Read the model definition and answer for the solid it produces. Units are mm, in the model's axes. Coordinates: 2 decimals unless noted, no trailing zeros. Write each loop counter-clockwise with the first axis right and the second up, starting at its lowest first coordinate (ties: lowest second). Pieces come first, ordered by that corner, then holes. Notation, with made-up numbers: (20, 17.25) -> (36, 17.25) arc R19 ccw to (36, 45.25) -> close; hole circle Ø2 at (-13, 54.5). An arc over 180 degrees is marked (long way). Use CSV: the item, a comma, the result in double quotes.
from build123d import *

# Parameters (mm, degrees)
EXTRUDE_1_DEPTH = 30


with BuildPart() as part:
    # 草图1 → 凸台-拉伸1 (new body)
    with BuildSketch(Plane.XY):
        with BuildLine():
            ThreePointArc((-15.712331266, 2.160724411), (-3.13309904, -15.547661374), (15.322874863, -4.093359222))
            ThreePointArc((15.322874863, -4.093359222), (78.436182954, -7.922682958), (139.19729869, -25.416687445))
            ThreePointArc((139.19729869, -25.416687445), (150.619110519, -21.552265679), (142.48119841, -12.654742004))
            ThreePointArc((142.48119841, -12.654742004), (43.215780263, 20.546958672), (-61.436350738, 18.570182304))
            ThreePointArc((-61.436350738, 18.570182304), (-69.151102392, 3.965497782), (-53.217470305, -0.385774624))
            ThreePointArc((-53.217470305, -0.385774624), (-34.831522248, 6.287119165), (-15.712331266, 2.160724411))
        make_face()
    extrude(amount=EXTRUDE_1_DEPTH)


solid = part.part
1. A cutting plane is placed at A-A (z = 26). Give the vertices of the cut face in (x, y).
Solutions:
outline,"(-61.44, 18.57) arc R10.58 ccw (long way) to (-53.22, -0.39) arc R35.34 cw to (-15.71, 2.16) arc R15.86 ccw to (15.32, -4.09) arc R288.34 cw to (139.2, -25.42) arc R7.2 ccw (long way) to (142.48, -12.65) arc R307.85 ccw to start"
2. For a pull along X with two mould halves and no side action, classify faces 1 (the cylindrical face through (44.67, 20.32, 14.79)), 2 (the flat face through (39, 5, 0)), 3 (the cylindrical face through (-35.108, 6.267, 14.79)) as pulls with the +X half, pulls with the -X half, needs draft (parallel to the pull), parting line crosses it, or undercut.
Solutions:
face 1,"parting line crosses it"
face 2,"needs draft"
face 3,"undercut"
3. Find the intervals of material crossed by line 1 along X through (y, z) = (0.5, 2.5); line 2 along Y through (x, z) = (130.5, 7); line 3 along Y through (x, z) = (110, 6), in increasing order.
Solutions:
line 1,"x = -66.73 to -51.94, -15.85 to 114.81"
line 2,"y = -22 to -6.54"
line 3,"y = -15.2 to 2.45"
4. A cutting plane is placed at C-C (y = 12). Give the vertices of the cut face in (x, z), and give its area (3 significant figures).
Solutions:
outline,"(-69.31, 0) -> (82.06, 0) -> (82.06, 30) -> (-69.31, 30) -> close"
area,"4,540 mm^2"
5. A cutting plane is placed at B-B (x = -46). Give the vertices of the cut face in (y, z).
Solutions:
outline,"(3.66, 0) -> (21.13, 0) -> (21.13, 30) -> (3.66, 30) -> close"
6. Each of these flat-tipped pins is pushed along its axis until it touches: pin 1 Ø6 at (x, z) = (7.5, 27) entering from -Y; pin 2 Ø3 at (x, z) = (-25.5, 24) entering from -Y; pin 3 Ø4 at (y, z) = (-8, 17.5) entering from -X. Where does it stop, or does it pass through?
Solutions:
pin 1,"stops at y = -15.21"
pin 2,"stops at y = 5.35"
pin 3,"stops at x = -14.68"
